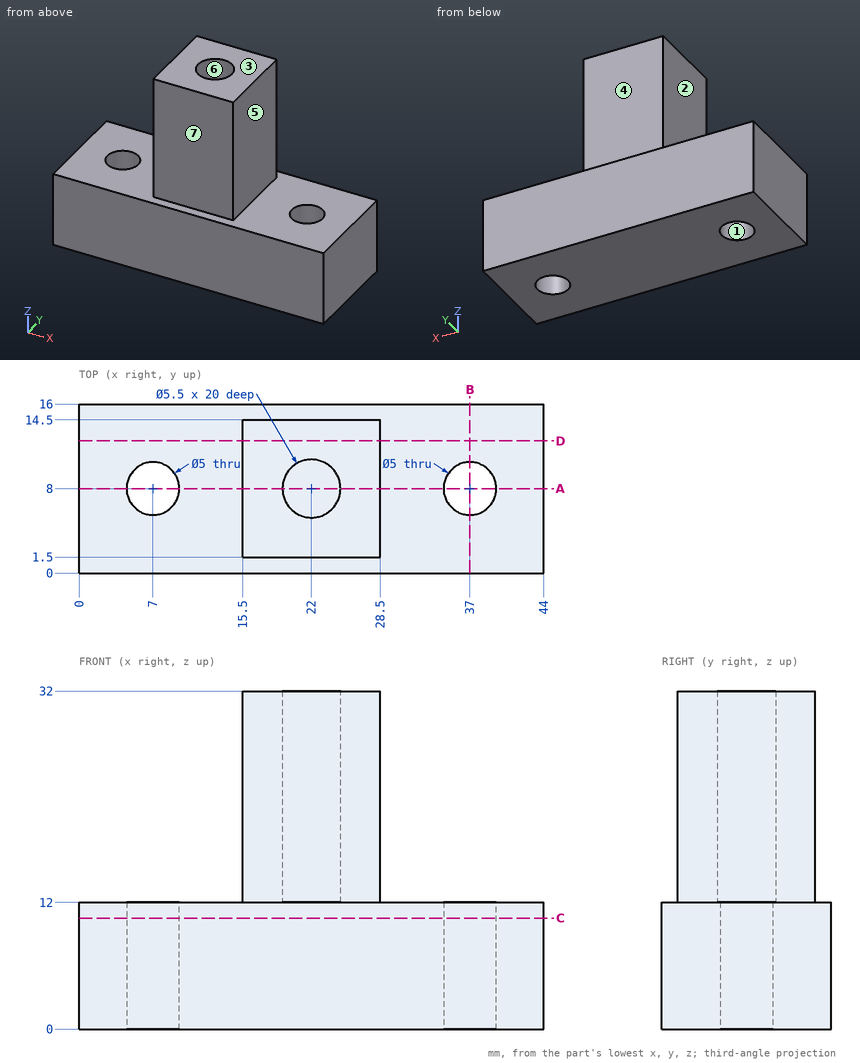
Can you work these out from the drawing? Everything is in mm from the part's minimum corner. A direction names the side the tool comes from. Coordinates: 2 decimals unless noted, no trailing zeros. Loops run counter-clockwise (first coordinate to the right, second up) from the corner with the lowest first, then second, coordinate; pieces in that order, holes last.
1) I need wall thicknesses on probe 1 along Y at (x, z) = (37, 4); probe 2 along Y at (x, z) = (22, 21); probe 3 along Z at (x, y) = (14, 4). Which ranges of each line are inside material? Lowest first, please.
2) Imagine slicing it at A-A on y = 8. List the corners of the cut face in (x, z) for me.
3) Imagine slicing it at D-D on y = 12.5. List the corners of the cut face in (x, z) for me.
4) Which directions (+Z, -Z, +X, -X, +Y, -Y) give clear straight access to the entire face, cutting with the end or side of a thin tool? Please do the marked faces 4, 5, 6 and 7.
5) Imagine slicing it at B-B on x = 37. List the corners of the cut face in (y, z) for me, plus the area to 3 significant figures.
6) For pin 1 (4 mm diameter, centred on x = 25, z = 19.5, fed in from -Y); pin 2 (1 mm diameter, centred on x = 29.5, y = 5.5, fed in from +Z); pin 3 (1.5 mm diameter, centred on x = 14, z = 15, fed in from +Y); pin 4 (4 mm diameter, centred on y = 2, z = 18, fed in from -X), each with a flat end and sliding along its axis, tell me the tip position at first contact or that it passes through.
7) Imagine slicing it at C-C on z = 10.5. List the corners of the cut face in (x, y) for me, plus the area to 3 significant figures.
8) Thinking about a two-plate mould opening in X: for the marked faces 1, 2 and 3, which applies, pulls with the +X half, pulls with the -X half, needs draft (parallel to the pull), parting line crosses it, or undercut?
Completed:
1. probe 1: y = 0 to 5.5, 10.5 to 16
1. probe 2: y = 1.5 to 5.25, 10.75 to 14.5
1. probe 3: z = 0 to 12
2. outline: (0, 0) - (4.5, 0) - (4.5, 12) - (0, 12) - close; (9.5, 0) - (34.5, 0) - (34.5, 12) - (28.5, 12) - (28.5, 32) - (24.75, 32) - (24.75, 12) - (19.25, 12) - (19.25, 32) - (15.5, 32) - (15.5, 12) - (9.5, 12) - close; (39.5, 0) - (44, 0) - (44, 12) - (39.5, 12) - close
3. outline: (0, 0) - (44, 0) - (44, 12) - (28.5, 12) - (28.5, 32) - (15.5, 32) - (15.5, 12) - (0, 12) - close
4. face 4: +Z, +X, -X, +Y
4. face 5: +Z, +X, +Y, -Y
4. face 6: +Z
4. face 7: +Z, +X, -X, -Y
5. outline: (0, 0) - (5.5, 0) - (5.5, 12) - (0, 12) - close; (10.5, 0) - (16, 0) - (16, 12) - (10.5, 12) - close
5. area: 132 mm2
6. pin 1: stops at y = 1.5
6. pin 2: stops at z = 12
6. pin 3: passes through
6. pin 4: stops at x = 15.5
7. outline: (0, 0) - (44, 0) - (44, 16) - (0, 16) - close; hole circle Ø5 at (7, 8); hole circle Ø5 at (37, 8)
7. area: 665 mm2
8. face 1: undercut
8. face 2: pulls with the -X half
8. face 3: needs draft
